```python
from build123d import *

# Parameters (mm, degrees)
SKETCH1_R               = 10
SKETCH1_R_2             = 0.8
SKETCH1_R_3             = 3.301767793
BOSS_EXTRUDE1_DEPTH     = 1.5
SKETCH2_R               = 10
BOSS_EXTRUDE2_DEPTH     = 9
SKETCH3_R               = 1.5
CUT_EXTRUDE1_DEPTH      = 1
CUT_EXTRUDE1_DEPTH_BACK = 10
FILLET1_R               = 5
SKETCH4_R               = 1.5
BOSS_EXTRUDE3_DEPTH     = 4
SKETCH5_W               = 43.786924739
SKETCH5_H               = 105.486682325
CUT_EXTRUDE2_DEPTH      = 5
CUT_EXTRUDE2_DEPTH_BACK = 10.0000001
CUT_EXTRUDE3_DEPTH      = 1
CUT_EXTRUDE3_DEPTH_BACK = 5


with BuildPart() as part:
    # Sketch1 → Boss-Extrude1 (new body)
    with BuildSketch(Plane(origin=(0, 0, 0), x_dir=(0, 0, -1), z_dir=(1, 0, 0))):
        with Locations((2.983378847, 10.826778074)):
            Circle(SKETCH1_R)
        with Locations((2.983378847, 18.576778074)):
            Circle(SKETCH1_R_2, mode=Mode.SUBTRACT)
        with Locations((2.983378847, 3.076778074)):
            Circle(SKETCH1_R_2, mode=Mode.SUBTRACT)
        with Locations((-3.266621153, 10.826778074)):
            Circle(SKETCH1_R_2, mode=Mode.SUBTRACT)
        with Locations((9.233378847, 10.826778074)):
            Circle(SKETCH1_R_2, mode=Mode.SUBTRACT)
        with Locations((2.983378847, 10.826778074)):
            Circle(SKETCH1_R_3, mode=Mode.SUBTRACT)
    extrude(amount=BOSS_EXTRUDE1_DEPTH)

    # Sketch2 → Boss-Extrude2 (add)
    with BuildSketch(Plane.ZY):
        with BuildLine():
            Line((-15.531923741, 95.891603494), (9.565166047, 95.891603494))
            Line((9.565166047, 95.891603494), (9.565166047, 10.826778074))
            ThreePointArc((9.565166047, 10.826778074), (-2.983378847, -1.721766821), (-15.531923741, 10.826778074))
            Line((-15.531923741, 10.826778074), (-15.531923741, 95.891603494))
        make_face()
        with Locations((-2.983378847, 10.826778074)):
            Circle(SKETCH2_R, mode=Mode.SUBTRACT)
    extrude(amount=-BOSS_EXTRUDE2_DEPTH)

    # Sketch3 → Cut-Extrude1 (cut, two sides)
    with BuildSketch(Plane(origin=(9, 0, 0), x_dir=(0, 0, -1), z_dir=(1, 0, 0))) as cut_extrude1_sk:
        with Locations((2.983378847, 90.473665847)):
            Circle(SKETCH3_R)
        with BuildLine():
            Line((-3.051129507, 36.150412664), (-3.051129507, 97.572569437))
            Line((-3.051129507, 97.572569437), (-16.389018159, 97.572569437))
            Line((-16.389018159, 97.572569437), (-16.389018159, 8.14109285))
            Line((-16.389018159, 8.14109285), (-9.565166047, 10.826778074))
            add(Edge.make_bspline(
                [(-9.565166047, 10.826778074), (-9.644230884, 15.122204253), (-6.916245701, 23.507010268), (-3.42826878, 31.561714956), (-3.051129507, 36.150412664)],
                knots=[0, 0, 0, 0, 0.482384809, 1, 1, 1, 1], degree=3))
        make_face()
        with BuildLine():
            Line((22.355775853, 8.14109285), (15.531923741, 10.826778074))
            add(Edge.make_bspline(
                [(15.531923741, 10.826778074), (15.610988578, 15.122204253), (12.883003395, 23.507010268), (9.395026474, 31.561714956), (9.017887201, 36.150412664)],
                knots=[0, 0, 0, 0, 0.482384809, 1, 1, 1, 1], degree=3))
            Line((9.017887201, 36.150412664), (9.017887201, 97.572569437))
            Line((9.017887201, 97.572569437), (22.355775853, 97.572569437))
            Line((22.355775853, 97.572569437), (22.355775853, 8.14109285))
        make_face()
    extrude(amount=CUT_EXTRUDE1_DEPTH, mode=Mode.SUBTRACT)
    extrude(cut_extrude1_sk.sketch, amount=-CUT_EXTRUDE1_DEPTH_BACK, mode=Mode.SUBTRACT)

    # Fillet1
    fillet1_edges = [part.edges().sort_by_distance(p)[0] for p in [
        (4.5, 95.891603494, 3.051129507),
        (4.5, 95.891603494, -9.017887201),
    ]]
    fillet(fillet1_edges, radius=FILLET1_R)

    # Sketch5 → Cut-Extrude2 (cut, two sides)
    with BuildSketch(Plane(origin=(9, 0, 0), x_dir=(0, 0, -1), z_dir=(1, 0, 0))) as cut_extrude2_sk:
        with Locations((-1.981744939, 44.563852974)):
            Rectangle(SKETCH5_W, SKETCH5_H)
    extrude(amount=CUT_EXTRUDE2_DEPTH, mode=Mode.SUBTRACT)
    extrude(cut_extrude2_sk.sketch, amount=-CUT_EXTRUDE2_DEPTH_BACK, mode=Mode.SUBTRACT)


with BuildPart() as body_2:
    # Sketch4 → Boss-Extrude3 (new body)
    with BuildSketch(Plane(origin=(9, 0, 0), x_dir=(0, 0, -1), z_dir=(1, 0, 0))):
        with BuildLine():
            Line((38.773588851, 85.849332764), (38.773588851, 10.849332764))
            ThreePointArc((38.773588851, 10.849332764), (34.779514456, 6.855258369), (30.785440062, 10.849332764))
            Line((30.785440062, 10.849332764), (30.785440062, 85.849332764))
            ThreePointArc((30.785440062, 85.849332764), (34.779514456, 89.843407159), (38.773588851, 85.849332764))
        make_face()
        with Locations((34.779514456, 85.849332764)):
            Circle(SKETCH4_R, mode=Mode.SUBTRACT)
        with Locations((34.779514456, 10.849332764)):
            Circle(SKETCH4_R, mode=Mode.SUBTRACT)
    extrude(amount=BOSS_EXTRUDE3_DEPTH)

    # Sketch6 → Cut-Extrude3 (cut, two sides)
    with BuildSketch(Plane(origin=(13, 0, 0), x_dir=(0, 0, -1), z_dir=(1, 0, 0))) as cut_extrude3_sk:
        with BuildLine():
            Line((32.368772821, 74.957140703), (32.368772821, 21.741524825))
            ThreePointArc((32.368772821, 21.741524825), (25.269119008, 14.641871012), (18.169465194, 21.741524825))
            Line((18.169465194, 21.741524825), (18.169465194, 74.957140703))
            ThreePointArc((18.169465194, 74.957140703), (25.269119008, 82.056794517), (32.368772821, 74.957140703))
        make_face()
        with BuildLine():
            Line((37.190256091, 74.957140703), (37.190256091, 21.741524825))
            ThreePointArc((37.190256091, 21.741524825), (44.289909905, 14.641871012), (51.389563719, 21.741524825))
            Line((51.389563719, 21.741524825), (51.389563719, 74.957140703))
            ThreePointArc((51.389563719, 74.957140703), (44.289909905, 82.056794517), (37.190256091, 74.957140703))
        make_face()
    extrude(amount=CUT_EXTRUDE3_DEPTH, mode=Mode.SUBTRACT)
    extrude(cut_extrude3_sk.sketch, amount=-CUT_EXTRUDE3_DEPTH_BACK, mode=Mode.SUBTRACT)


solid = body_2.part
```
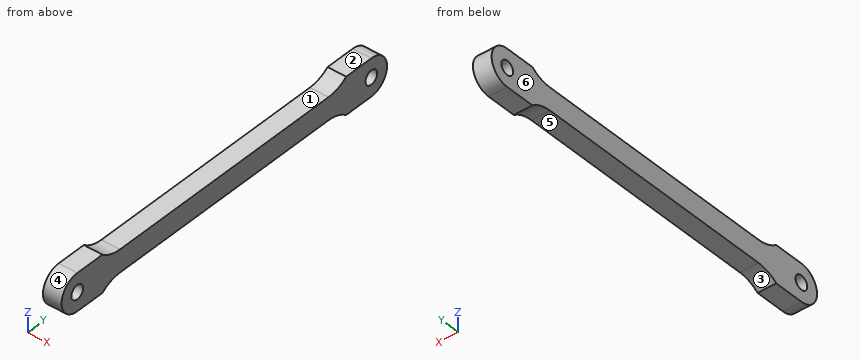
The listing builds one solid part. Answer for the finished solid, in the listing's coordinates (mm). Face numbers are marked on the shaded views. A direction names the side the tool comes from. Round coordinates to 2 decimals unless told otherwise and drop trailing zeros. Write each loop counter-clockwise with the first axis right and the second up, starting at its lowest first coordinate (ties: lowest second). Pieces come first, ordered by that corner, then holes. Notation, with made-up numbers: (-26, 51) -> (32, 51) arc R19 cw to (32, 70) -> close; hole circle Ø3 at (12.25, -3). An arc over 180 degrees is marked (long way). Write item = value, one per line.
1) Section A-A on z = -38 is taken. Write down the section's boundary in (x, y), plus the area to 3 significant figures.
Check values:
outline = (9, 8.49) -> (13, 8.49) -> (13, 18.45) -> (9, 18.45) -> close; (9, 78.25) -> (13, 78.25) -> (13, 88.21) -> (9, 88.21) -> close
area = 79.7 mm²
2) Section C-C on z = -34 is taken. Write down the section's boundary in (x, y), plus the area to 3 significant figures.
Check values:
outline = (9, 6.93) -> (13, 6.93) -> (13, 9.57) -> (9, 9.57) -> close; (9, 12.13) -> (13, 12.13) -> (13, 84.57) -> (9, 84.57) -> close; (9, 87.13) -> (13, 87.13) -> (13, 89.77) -> (9, 89.77) -> close
area = 311 mm²
3) Given pin 1 (1.2 mm diameter, centred on x = 11, y = 36.5, fed in from -Z); pin 2 (1.5 mm diameter, centred on x = 12.5, y = 72, fed in from +Z); pin 3 (1.8 mm diameter, centred on y = 10.85, z = -34.78, fed in from +X), each flat-ended and moving along its own axis, determine where each tip first touches the part or whether it passes through.
Check values:
pin_1 = -37.19
pin_2 = -32.37
pin_3 = through
4) For a pull along Y with two mould halves and no side action, classify the marked faces 4, 5 and 6 as released by +Y, released by -Y, zero draft, split by the parting line, or undercut.
Check values:
face_4 = released by -Y
face_5 = undercut
face_6 = zero draft
5) Section B-B on x = 11.8 is taken. Write down the section's boundary in (y, z).
Check values:
outline = (10.85, -38.77) -> (17.27, -38.77) arc R7.1 cw to (21.74, -37.19) -> (74.96, -37.19) arc R7.1 cw to (79.43, -38.77) -> (85.85, -38.77) arc R3.99 ccw to (85.85, -30.79) -> (79.43, -30.79) arc R7.1 cw to (74.96, -32.37) -> (21.74, -32.37) arc R7.1 cw to (17.27, -30.79) -> (10.85, -30.79) arc R3.99 ccw to start; hole circle Ø3 at (10.85, -34.78); hole circle Ø3 at (85.85, -34.78)
6) Section D-D on y = 59 is taken. Write down the section's boundary in (x, z).
Check values:
outline = (9, -37.19) -> (13, -37.19) -> (13, -32.37) -> (9, -32.37) -> close
7) Straight lines are drawn through the part: line 1 along Y through (x, z) = (9.8, -34.5); line 2 along Z through (x, y) = (12.55, 26.5); line 3 along Y through (x, z) = (11.5, -35.75). For each, find the intervals that lie inside material, in ascending order. Write a range as [from, to].
Check values:
line_1 = [6.87, 9.38], [12.32, 84.38], [87.32, 89.83]
line_2 = [-37.19, -32.37]
line_3 = [6.97, 9.71], [11.99, 84.71], [86.99, 89.72]
8) Which of the six approach directions +Z, -Z, +X, -X, +Y, -Y give full straight-line access (tool end or side, diameter ignored) to the marked faces 1, 2 and 3?
Check values:
face_1 = +Z, +X, -X
face_2 = +Z, +X, -X, +Y, -Y
face_3 = -Z, +X, -X
